```python
from build123d import *

# Parameters (mm, degrees)
SKETCH1_W            = 35
SKETCH1_H            = 12
BOSS_EXTRUDE1_DEPTH  = 6
SKETCH3_W            = 19.5
SKETCH3_H            = 4.75
BOSS_EXTRUDE2_DEPTH  = 12
M6_CLEARANCE_HOLE1_D = 6.4
CHAMFER4_SIZE        = 1


with BuildPart() as part:
    # Sketch1 → Boss-Extrude1 (new, symmetric)
    with BuildSketch(Plane.XY):
        Rectangle(SKETCH1_W, SKETCH1_H)
    extrude(amount=BOSS_EXTRUDE1_DEPTH, both=True)

    # Sketch3 → Boss-Extrude2 (add)
    with BuildSketch(Plane(origin=(0, 6, 0), x_dir=(1, 0, 0), z_dir=(0, 1, 0))):
        with Locations((0, 8.375)):
            Rectangle(SKETCH3_W, SKETCH3_H)
    extrude(amount=-BOSS_EXTRUDE2_DEPTH)

    # M6 Clearance Hole1 (through all)
    with Locations(Plane(origin=(0, 6, 0), x_dir=(1, 0, 0), z_dir=(0, 1, 0))):
        with Locations((-7.5, 0), (7.5, 0)):
            Hole(M6_CLEARANCE_HOLE1_D / 2)

    # Chamfer4
    chamfer4_edges = [part.edges().sort_by_distance(p)[0] for p in [
        (-17.5, 0, 6),
        (0, -6, 6),
        (-9.75, 0, -10.75),
        (9.75, 0, -10.75),
        (0, 6, -10.75),
        (0, -6, -10.75),
        (17.5, 0, 6),
        (-17.5, 0, -6),
        (17.5, 0, -6),
        (17.5, -6, 0),
        (-17.5, -6, 0),
        (-17.5, 6, 0),
        (17.5, 6, 0),
        (0, 6, 6),
    ]]
    chamfer(chamfer4_edges, length=CHAMFER4_SIZE)


solid = part.part
```
Can you work these out from the model? Positions are in its coordinate system, mm. A direction names the side the tool comes from. Give positions to 0.01 mm unless a question says otherwise; leave off trailing zeros. Loops run counter-clockwise (first coordinate to the right, second up) from the corner with the lowest first, then second, coordinate; pieces in that order, holes last. Notation, with made-up numbers: M 53,-30.75 L 109,-30.75 A29 cw 109,-1.75 Z; hole C 52,27.5 d2. An arc over 180 degrees is marked long. Use CSV: the item, a comma, the result in double quotes. Start each with the question number.
1. For P1, Ø1.1, axis at y = -1.5, z = -7.5, coming from the +X side; P2, Ø1, axis at x = -12.5, y = 1, coming from the -Z side; P3, Ø1.9, axis at y = 1.5, z = -7, coming from the -X side, each with a flat end and sliding along its axis, tell me the tip position at first contact or that it passes through.
2. Imagine slicing it at A-A, the plane z = 0. Write out the boundary of the cut face in (x, y), plus the area to 3 significant figures.
3. Imagine slicing it at B-B, the plane x = -7.5. Write out the boundary of the cut face in (y, z).
4. If I drill on L1, parallel to Z at x = 7.5, y = -1; L2, parallel to X at y = -5.5, z = 2; L3, parallel to X at y = 1.5, z = 0.25, over which ranges is the centre line in solid material (lowest first)?
5. If we mould it in two halves opening along Z, with no side actions, what happens to faces 1 (the face through (-10.456, -0.084, 1.226)), 2 (the face through (17, -5.5, -0.6)), 3 (the face through (-0.2, -5.5, 5.5))? For each: released by +Z, released by -Z, zero draft, split by the parting line, or undercut.
6. Imagine slicing it at D-D, the plane x = -14. Write out the boundary of the cut face in (y, z).
7. Imagine slicing it at C-C, the plane y = 4.5. Write out the boundary of the cut face in (x, z).
8. On a 3-axis mill with a long thin cutter (end or side, diameter ignored), from which of +Z, -Z, +X, -X, +Y, -Y can I reach the whole of each face in a straight line? I mean faces 4 (the face through (9.75, 0, -8)), 5 (the face through (17, 5.5, -0.4)), 6 (the face through (-9.75, 0, -8)). Say none if no direction works.
Response values:
1,P1,"x = 9.75"
1,P2,"z = -6"
1,P3,"x = -9.75"
2,outline,"M -17.5,-5 L -16.5,-6 L -10.7,-6 L -10.7,6 L -16.5,6 L -17.5,5 Z; M -4.3,-6 L 4.3,-6 L 4.3,6 L -4.3,6 Z; M 10.7,-6 L 16.5,-6 L 17.5,-5 L 17.5,5 L 16.5,6 L 10.7,6 Z"
2,area,"264 mm^2"
3,outline,"M -6,-9.75 L -5,-10.75 L 5,-10.75 L 6,-9.75 L 6,-3.2 L -6,-3.2 Z; M -6,3.2 L 6,3.2 L 6,5 L 5,6 L -5,6 L -6,5 Z"
4,L1,"-10.75 to -3.2, 3.2 to 6"
4,L2,"-17 to -10, -5 to 5, 10 to 17"
4,L3,"-17.5 to -10.69, -4.31 to 4.31, 10.69 to 17.5"
5,face 1,"undercut"
5,face 2,"zero draft"
5,face 3,"released by +Z"
6,outline,"M -6,-6 L 6,-6 L 6,5 L 5,6 L -5,6 L -6,5 Z"
7,outline,"M -17.5,-5 L -16.5,-6 L -9.75,-6 L -9.75,-9.75 L -8.75,-10.75 L 8.75,-10.75 L 9.75,-9.75 L 9.75,-6 L 16.5,-6 L 17.5,-5 L 17.5,5 L 16.5,6 L -16.5,6 L -17.5,5 Z; hole C -7.5,0 d6.4; hole C 7.5,0 d6.4"
8,face 4,"-Z, +X, +Y, -Y"
8,face 5,"+Z, -Z, +X, +Y"
8,face 6,"-Z, -X, +Y, -Y"
